Can you work these out from the model? Positions are in its coordinate system, mm. A direction names the side the tool comes from. Give positions to 0.01 mm unless a question says otherwise; leave off trailing zeros. Loops run counter-clockwise (first coordinate to the right, second up) from the corner with the lowest first, then second, coordinate; pieces in that order, holes last. Notation, with made-up numbers: (67, 61.5) -> (74, 61.5) arc R19 ccw to (74, 79.5) -> close; hole circle Ø7 at (79, 37). An arc over 180 degrees is marked (long way). Return JSON: item names as keys, results as strings. Group by question number.
Q1. Suppose I cut it at B-B, the plane y = 18.5. Please give me the cut outline in (x, z).
Q2. Thinking about a two-plate mould opening in Z: for faces 1 (the flat face through (43.642, 3, 24)), 2 (the flat face through (6, -21, 23.532)), 3 (the cylindrical face through (-35.884, 1.515, 28.062)), 4 (the cylindrical face through (48.125, 1.515, 28.062)), which applies, pulls with the +Z half, pulls with the -Z half, needs draft (parallel to the pull), parting line crosses it, or undercut?
Q3. Suppose I cut it at D-D, the plane z = 11. Please give me the cut outline in (x, y), and give its area (3 significant figures).
Q4. Suppose I cut it at C-C, the plane z = 42. Please give me the cut outline in (x, y), and give its area (3 significant figures).
Q5. Which directions (+Z, -Z, +X, -X, +Y, -Y) give clear straight access to the entire face, cutting with the end or side of a thin tool? Please do faces 5 (the flat face through (5, -18.113, 19)), 6 (the flat face through (6, 27, 23.532)), 7 (the flat face through (6, -21, 0)).
Q6. I need wall thicknesses on line 1 along Y through (x, z) = (32, 38.5); line 2 along X through (y, z) = (-7.5, 17.5); line 3 along X through (y, z) = (-21.5, 41.5). Which ranges of each line are inside material? Lowest first, please. Write a range as [from, to].
Q7. Will these pins go through, and if not, where does the flat tip stop? pin 1 (2 mm diameter, centred on x = -4.5, y = -22.5, fed in from +Z); pin 2 (14 mm diameter, centred on y = 2.85, z = 34.09, fed in from -X).
Q8. Suppose I cut it at A-A, the plane x = -29.5. Please give me the cut outline in (y, z).
```python
from build123d import *

# Parameters (mm, degrees)
F0_W     = 92.417967
F0_H     = 55.051444
F1_DEPTH = 47.244
F2_W     = 75.588774
F2_H     = 42.215616
F3_DEPTH = 47.245
F4_W     = 50.487596
F4_H     = 23.711647
F5_DEPTH = 55.052444
F6_R     = 6.170698
F7_DEPTH = 92.418967


with BuildPart() as f1:
    # F0 (on Top) → F1 (new body)
    with BuildSketch(Plane.XY):
        with Locations((6.275294, 2.852407)):
            Rectangle(F0_W, F0_H)
    extrude(amount=F1_DEPTH)

    # F2 (on face) → F3 (cut, through all)
    with BuildSketch(Plane.XY.offset(47.244)):
        with Locations((5.847434, 2.995027)):
            Rectangle(F2_W, F2_H)
    extrude(amount=-F3_DEPTH, mode=Mode.SUBTRACT)

    # F4 (on face) → F5 (cut, through all)
    with BuildSketch(Plane.XZ.offset(24.673315)):
        with Locations((6.703155, 35.388177)):
            Rectangle(F4_W, F4_H)
    extrude(amount=-F5_DEPTH, mode=Mode.SUBTRACT)

    # F6 (on face) → F7 (cut, through all)
    with BuildSketch(Plane.YZ.offset(52.484278)):
        with Locations((2.852408, 34.086257)):
            Circle(F6_R)
    extrude(amount=-F7_DEPTH, mode=Mode.SUBTRACT)


solid = f1.part
```
Ans:
{
 "1": {"outline": "(-39.93, 0) -> (-31.95, 0) -> (-31.95, 47.24) -> (-39.93, 47.24) -> close; (43.64, 0) -> (52.48, 0) -> (52.48, 47.24) -> (43.64, 47.24) -> close"},
 "2": {"face 1": "needs draft", "face 2": "pulls with the +Z half", "face 3": "undercut", "face 4": "undercut"},
 "3": {"outline": "(-39.93, -24.67) -> (52.48, -24.67) -> (52.48, 30.38) -> (-39.93, 30.38) -> close; hole (-31.95, -18.11) -> (43.64, -18.11) -> (43.64, 24.1) -> (-31.95, 24.1) -> close", "area": "1,900 mm^2"},
 "4": {"outline": "(-39.93, -24.67) -> (-18.54, -24.67) -> (-18.54, -18.11) -> (-31.95, -18.11) -> (-31.95, 24.1) -> (-18.54, 24.1) -> (-18.54, 30.38) -> (-39.93, 30.38) -> close; (31.95, -24.67) -> (52.48, -24.67) -> (52.48, 30.38) -> (31.95, 30.38) -> (31.95, 24.1) -> (43.64, 24.1) -> (43.64, -18.11) -> (31.95, -18.11) -> close", "area": "1,250 mm^2"},
 "5": {"face 5": "+Z, -Z", "face 6": "+Z, +Y, -Y", "face 7": "-Z, +X, -X, +Y, -Y"},
 "6": {"line 1": "y = [-24.67, -18.11], [24.1, 30.38]", "line 2": "x = [-39.93, -31.95], [43.64, 52.48]", "line 3": "x = [-39.93, -18.54], [31.95, 52.48]"},
 "7": {"pin 1": "stops at z = 23.53", "pin 2": "stops at x = -39.93"},
 "8": {"outline": "(-24.67, 0) -> (-18.11, 0) -> (-18.11, 47.24) -> (-24.67, 47.24) -> close; (24.1, 0) -> (30.38, 0) -> (30.38, 47.24) -> (24.1, 47.24) -> close"}
}
